Geometry: final body of the model. Coordinates: model frame, mm. A direction names the side the tool comes from. Coordinates: 2 decimals unless noted, no trailing zeros. Write each loop counter-clockwise with the first axis right and the second up, starting at its lowest first coordinate (ties: lowest second). Pieces come first, ordered by that corner, then holes. Notation, with made-up numbers: (47.5, -24) - (99.5, -24) arc R21 cw to (99.5, -20) - close; hole circle Ø9 at (80, 77). An arc over 180 degrees is marked (long way). Put each result on its own line as item: value.
```python
from build123d import *

# Parameters (mm, degrees)
ESQUISSE1_W        = 5
ESQUISSE1_H        = 5
BOSS_EXTRU_1_DEPTH = 5


with BuildPart() as part:
    # Esquisse1 → Boss.-Extru.1 (new body)
    with BuildSketch(Plane.XY):
        Polygon((-70, 144), (-80, 144), (-80, 0), (-70, 0), (-70, -5), (-70, -12), (-65, -12), (-65, -10), (-66.5, -10), (-66.5, -5), (-65, -5), (-65, 0), (-60, 0), (-55, 0), (-55, -5), (-53.5, -5), (-53.5, -10), (-55, -10), (-55, -12), (-50, -12), (-50, -5), (-50, 0), (-30, 0), (-30, -5), (-25, -5), (-25, 0), (-20, 0), (-15, 0), (-15, -5), (-10, -5), (-10, 0), (10, 0), (10, -5), (15, -5), (15, 0), (20, 0), (25, 0), (25, -5), (30, -5), (30, 0), (50, 0), (50, -5), (50, -12), (55, -12), (55, -10), (53.5, -10), (53.5, -5), (55, -5), (55, 0), (60, 0), (65, 0), (65, -5), (66.5, -5), (66.5, -10), (65, -10), (65, -12), (70, -12), (70, -5), (70, 0), (80, 0), (80, 144), (70, 144), (70, 149), (70, 156), (65, 156), (65, 154), (66.5, 154), (66.5, 149), (65, 149), (65, 144), (60, 144), (55, 144), (55, 149), (53.5, 149), (53.5, 154), (55, 154), (55, 156), (50, 156), (50, 149), (50, 144), (30, 144), (30, 149), (25, 149), (25, 144), (20, 144), (15, 144), (15, 149), (10, 149), (10, 144), (-10, 144), (-10, 149), (-15, 149), (-15, 144), (-20, 144), (-25, 144), (-25, 149), (-30, 149), (-30, 144), (-50, 144), (-50, 149), (-50, 156), (-55, 156), (-55, 154), (-53.5, 154), (-53.5, 149), (-55, 149), (-55, 144), (-60, 144), (-65, 144), (-65, 149), (-66.5, 149), (-66.5, 154), (-65, 154), (-65, 156), (-70, 156), (-70, 149), align=None)
        with Locations((-74.5, 4.5)):
            Rectangle(ESQUISSE1_W, ESQUISSE1_H, mode=Mode.SUBTRACT)
        with Locations((-74.5, 19.5)):
            Rectangle(ESQUISSE1_W, ESQUISSE1_H, mode=Mode.SUBTRACT)
        with Locations((-74.5, 44.5)):
            Rectangle(ESQUISSE1_W, ESQUISSE1_H, mode=Mode.SUBTRACT)
        with Locations((-74.5, 59.5)):
            Rectangle(ESQUISSE1_W, ESQUISSE1_H, mode=Mode.SUBTRACT)
        with Locations((74.5, 4.5)):
            Rectangle(ESQUISSE1_W, ESQUISSE1_H, mode=Mode.SUBTRACT)
        with Locations((74.5, 19.5)):
            Rectangle(ESQUISSE1_W, ESQUISSE1_H, mode=Mode.SUBTRACT)
        with Locations((74.5, 44.5)):
            Rectangle(ESQUISSE1_W, ESQUISSE1_H, mode=Mode.SUBTRACT)
        with Locations((74.5, 59.5)):
            Rectangle(ESQUISSE1_W, ESQUISSE1_H, mode=Mode.SUBTRACT)
        with Locations((-74.5, 84.5)):
            Rectangle(ESQUISSE1_W, ESQUISSE1_H, mode=Mode.SUBTRACT)
        with Locations((-74.5, 99.5)):
            Rectangle(ESQUISSE1_W, ESQUISSE1_H, mode=Mode.SUBTRACT)
        with Locations((-74.5, 124.5)):
            Rectangle(ESQUISSE1_W, ESQUISSE1_H, mode=Mode.SUBTRACT)
        with Locations((-74.5, 139.5)):
            Rectangle(ESQUISSE1_W, ESQUISSE1_H, mode=Mode.SUBTRACT)
        with Locations((74.5, 84.5)):
            Rectangle(ESQUISSE1_W, ESQUISSE1_H, mode=Mode.SUBTRACT)
        with Locations((74.5, 99.5)):
            Rectangle(ESQUISSE1_W, ESQUISSE1_H, mode=Mode.SUBTRACT)
        with Locations((74.5, 124.5)):
            Rectangle(ESQUISSE1_W, ESQUISSE1_H, mode=Mode.SUBTRACT)
        with Locations((74.5, 139.5)):
            Rectangle(ESQUISSE1_W, ESQUISSE1_H, mode=Mode.SUBTRACT)
    extrude(amount=BOSS_EXTRU_1_DEPTH)


solid = part.part
```
1. Set-up query: faces 1 (the flat face through (50, -6, 2)), 2 (the flat face through (52, -12, 2)), 3 (the flat face through (74, 87, 2)). Return all of +Z, -Z, +X, -X, +Y, -Y with unobstructed straight access to the full face (end or side cutting, diameter ignored); none if empty.
Answer below:
face 1: +Z, -Z, -Y
face 2: +Z, -Z, +X, -X, -Y
face 3: +Z, -Z
2. Mould query, pull axis X, two halves, no side actions, for faces 4 (the flat face through (-67, 156, 2)), 5 (the flat face through (-15, -2, 2)). Classes: +X half, -X half, draft (parallel to the pull), parting line (faces both ways), or undercut.
Answer below:
face 4: draft
face 5: undercut
3. Section query A-A (z = 1.75). Count the separate pieces of the cut face and the enclosed holes in it, then the cut area to 3 significant figures.
Answer below:
separate pieces: 1
enclosed holes: 16
area: 23,300 mm²
4. Ray query, probe 1 along X at (y, z) = (126.5, 4.65); probe 2 along Y at (x, z) = (29, 0.7); probe 3 along Y at (x, z) = (42.5, 3). Return the intervals inside material, ascending. Write a range as from..to.
Answer below:
probe 1: x = -80..-77, -72..72, 77..80
probe 2: y = -5..149
probe 3: y = 0..144
5. Section query B-B (x = 23). Return loops of the section in (y, z), then the cut area to 3 significant figures.
Answer below:
outline: (0, 0) - (144, 0) - (144, 5) - (0, 5) - close
area: 720 mm²
6. Pin query (flat end, axial travel): pin 1 Ø2.5 at (y, z) = (146, 3) entering from -X; pin 2 Ø2.5 at (y, z) = (-2, 1.5) entering from +X; pin 3 Ø2.5 at (x, z) = (-74, 2.5) entering from +Y. Return the tip coordinate at first contact, or that it passes through.
Answer below:
pin 1: stops at x = -70
pin 2: stops at x = 70
pin 3: stops at y = 144
